For this review, take the finished solid that the model builds, in its own axes (mm). Face numbers are marked on the shaded views. Give positions to 0.01 mm unless a question says otherwise; leave off trailing zeros. Write each loop counter-clockwise with the first axis right and the second up, starting at its lowest first coordinate (ties: lowest second). Pieces come first, ordered by that corner, then holes.
Q1. We need section C-C (x = -48). Write out the cut boundary in (y, z), then the cut area to 3 significant figures.
Q2. For line 1 (X direction, y = -2.75, z = -23.5); line 2 (X direction, y = -7.75, z = -36); line 3 (Z direction, x = 31.5, y = -10.25), list the stretches that pass through material, from the lowest coordinate up.
Q3. We need section D-D (z = -23). Write out the cut boundary in (x, y).
Q4. We need section A-A (z = -31). Write out the cut boundary in (x, y).
Q5. Insertion check: P1, Ø1, axis at x = -50, y = -1.5, coming from the -Z side; P2, Ø2, axis at y = -10.5, z = -31, coming from the +X side. Each pin has a flat end and moves straight along its axis. Give the tip position at first contact, or say it passes through.
Q6. Mouldability with a two-part tool opening along X and no side actions: class the marked faces 1, 2 and 3 as released by +X, released by -X, zero draft, split by the parting line, or undercut.
```python
from build123d import *

# Parameters (mm, degrees)
F1_DEPTH = 12.7


# Not quite as in the source:
# - ends of sketch curves that miss each other by under 0.0002 mm in the source are joined


with BuildPart() as f1:
    # F0 (on Front) → F1 (new body)
    with BuildSketch(Plane.XZ):
        with BuildLine():
            Line((90.4875, -9.1365433148), (-90.4875, -9.1365433148))
            Line((-90.4875, -9.1365433148), (-90.4875, -18.6488433148))
            ThreePointArc((-90.4875, -18.6488433148), (-69.1593908483, -27.4832345546), (-60.3249986632, -48.8113433148))
            ThreePointArc((-60.3249986632, -48.8113433148), (-30.1625, -18.6615433148), (-2.6737e-06, -48.8113433154))
            ThreePointArc((-2.6737e-06, -48.8113433154), (30.1625, -18.6488433148), (60.325, -48.8113433148))
            ThreePointArc((60.325, -48.8113433148), (69.1593917125, -27.4832350273), (90.4875, -18.6488433148))
            Line((90.4875, -18.6488433148), (90.4875, -9.1365433148))
        make_face()
    extrude(amount=F1_DEPTH)


solid = f1.part
```
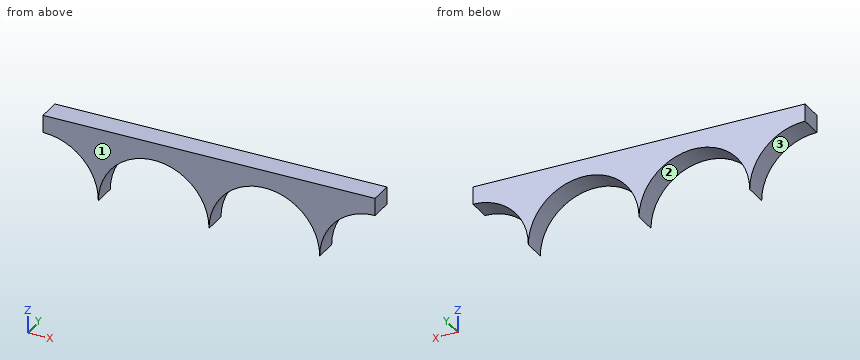
Computed:
1. outline: (-12.7, -24.5) - (0, -24.5) - (0, -9.14) - (-12.7, -9.14) - close
1. area: 195 mm2
2. line 1: x = -74.08 to -46.55, -13.78 to 13.76, 46.57 to 74.08
2. line 2: x = -63.18 to -57.46, -2.86 to 2.86, 57.47 to 63.18
2. line 3: z = -18.68 to -9.14
3. outline: (-74.88, -12.7) - (-45.75, -12.7) - (-45.75, 0) - (-74.88, 0) - close; (-14.58, -12.7) - (14.56, -12.7) - (14.56, 0) - (-14.58, 0) - close; (45.77, -12.7) - (74.88, -12.7) - (74.88, 0) - (45.77, 0) - close
4. outline: (-66.15, -12.7) - (-54.5, -12.7) - (-54.5, 0) - (-66.15, 0) - close; (-5.83, -12.7) - (5.82, -12.7) - (5.82, 0) - (-5.83, 0) - close; (54.5, -12.7) - (66.15, -12.7) - (66.15, 0) - (54.5, 0) - close
5. P1: stops at z = -26.55
5. P2: stops at x = 66.91
6. face 1: zero draft
6. face 2: undercut
6. face 3: released by -X
